from build123d import *

# Parameters (mm, degrees)
F1_DEPTH = 100
F2_R     = 10
F3_R     = 5
F3_R_2   = 8
F4_DEPTH = 60.001


with BuildPart() as f1:
    # F0 (on Front) → F1 (new body)
    with BuildSketch(Plane.XZ):
        Polygon((0, 15), (0, 0), (70, 0), (60, 40), (20, 40), (10, 60), (-20, 60), (-20, 25), align=None)
    extrude(amount=-F1_DEPTH)

    # F2
    f2_edges = [f1.edges().sort_by_distance(p)[0] for p in [
        (20, 50, 40),
        (0, 50, 15),
    ]]
    fillet(f2_edges, radius=F2_R)

    # F3 (on face) → F4 (cut, through all)
    with BuildSketch(Plane.XY.offset(60)):
        with Locations((0, 65)):
            Circle(F3_R)
        with Locations((45, 40)):
            Circle(F3_R_2)
    extrude(amount=-F4_DEPTH, mode=Mode.SUBTRACT)


solid = f1.part
The model under review builds one solid part; all positions refer to its coordinate system, in mm. A direction names the side the tool comes from. Round coordinates to 2 decimals unless told otherwise and drop trailing zeros. Loops run counter-clockwise (first coordinate to the right, second up) from the corner with the lowest first, then second, coordinate; pieces in that order, holes last. Notation, with made-up numbers: M 85.5,39 L 115.5,39 A25 cw 115.5,66 Z; hole C -5,-25 d9. An arc over 180 degrees is marked long. Answer as CSV lines item,"result".
1. Insertion check: pin 1 Ø4 at (y, z) = (10.5, 8.5) entering from -X; pin 2 Ø2.5 at (y, z) = (19, 5.5) entering from -X; pin 3 Ø5 at (y, z) = (27, 23) entering from +X (3 decimals). Each pin has a flat end and moves straight along its axis. Give the tip position at first contact, or say it passes through.
Outcome:
pin 1,"stops at x = -0.14"
pin 2,"stops at x = 0"
pin 3,"stops at x = 64.875"
2. Draft analysis for pull direction Y (two halves, no side actions). For faces 4 (the face through (24, 0, 24)), 5 (the face through (-5, 49, 60)), 6 (the face through (39.1, 45.4, 20.3)), state which applies: pulls with the +Y half, pulls with the -Y half, needs draft (parallel to the pull), parting line crosses it, or undercut.
Outcome:
face 4,"pulls with the -Y half"
face 5,"needs draft"
face 6,"undercut"
3. We need section D-D (y = 79.5). Give the boundary of the cut face in (x, z), plus the area to 3 significant figures.
Outcome:
outline,"M -20,25 L -5.53,17.76 A10 cw 0,8.82 L 0,0 L 70,0 L 60,40 L 26.18,40 A10 cw 17.24,45.53 L 10,60 L -20,60 Z"
area,"3,710 mm2"
4. For faces 1 (the face through (0, 30, 4)), 2 (the face through (24, 100, 24)), 3 (the face through (43, 49, 40)), list the 3-axis set-ups (+Z, -Z, +X, -X, +Y, -Y) from which the entire face can be reached by the end or side of a thin tool; tool diameter is ignored.
Outcome:
face 1,"-Z, -X, +Y, -Y"
face 2,"+Z, -Z, +X, -X, +Y"
face 3,"+Z, +X, +Y, -Y"
5. We need section B-B (y = 40). Give the boundary of the cut face in (x, z).
Outcome:
outline,"M -20,25 L -5.53,17.76 A10 cw 0,8.82 L 0,0 L 37,0 L 37,40 L 26.18,40 A10 cw 17.24,45.53 L 10,60 L -20,60 Z; M 53,0 L 70,0 L 60,40 L 53,40 Z"
6. To check wall thickness, follow L1, parallel to Y at x = -0.5, z = 49; L2, parallel to Z at x = 54, y = 60; L3, parallel to X at y = 65, z = 24. State the ranges of each line that lie inside material, in increasing order. Write a range as [from, to].
Outcome:
L1,"y = [0, 60.03], [69.97, 100]"
L2,"z = [0, 40]"
L3,"x = [-18, -5], [5, 64]"
7. We need section A-A (x = 45). Give the boundary of the cut face in (y, z).
Outcome:
outline,"M 0,0 L 32,0 L 32,40 L 0,40 Z; M 48,0 L 100,0 L 100,40 L 48,40 Z"
8. We need section C-C (z = 35). Give the boundary of the cut face in (x, y).
Outcome:
outline,"M -20,0 L 61.25,0 L 61.25,100 L -20,100 Z; hole C 0,65 d10; hole C 45,40 d16"
